The drawing under review shows one solid part. Ordinate dimensions are in mm from its lowest x, y, z. A direction names the side the tool comes from. Give positions to 0.01 mm unless a question says otherwise; leave off trailing zeros. Order: outer loops, then holes, each group sorted by start corner. A loop starts at its lowest first (then second) coordinate and runs counter-clockwise, first axis right, second up. Notation, with made-up numbers: (78, -23.5) -> (129, -23.5) arc R18 ccw to (129, -17.5) -> close; hole circle Ø9 at (79.5, 40). An arc over 180 degrees is marked (long way). Return JSON: item names as keys, results as strings. Group by question number.
1) For the marked faces 1, 2 and 3, list the 3-axis set-ups (+Z, -Z, +X, -X, +Y, -Y) from which the entire face can be reached by the end or side of a thin tool; tool diameter is ignored.
2) To check wall thickness, follow line 1 along X through (y, z) = (6.5, 33); line 2 along X through (y, z) = (16, 32); line 3 along Y through (x, z) = (53, 24). State the ranges of each line that lie inside material, in increasing order.
3) Add section B-B (x = 33). State how many separate pieces and enclosed holes the cut face has, then the cut area to 3 significant figures.
4) Add section A-A (y = 6.5). Give the boundary of the cut face in (x, z).
5) Insertion check: P1, Ø2, axis at y = 21, z = 51.5, coming from the +X side; P2, Ø6, axis at x = 55, y = 16.5, coming from the -Z side; P3, Ø6, axis at x = 41.5, y = 10.5, coming from the +Z side. Each pin has a flat end and moves straight along its axis. Give the tip position at first contact, or say it passes through.
6) The part is to be moulded in two halves that separate along X. For the marked faces 4, 5 and 6, say which applies: released by +X, released by -X, zero draft, split by the parting line, or undercut.
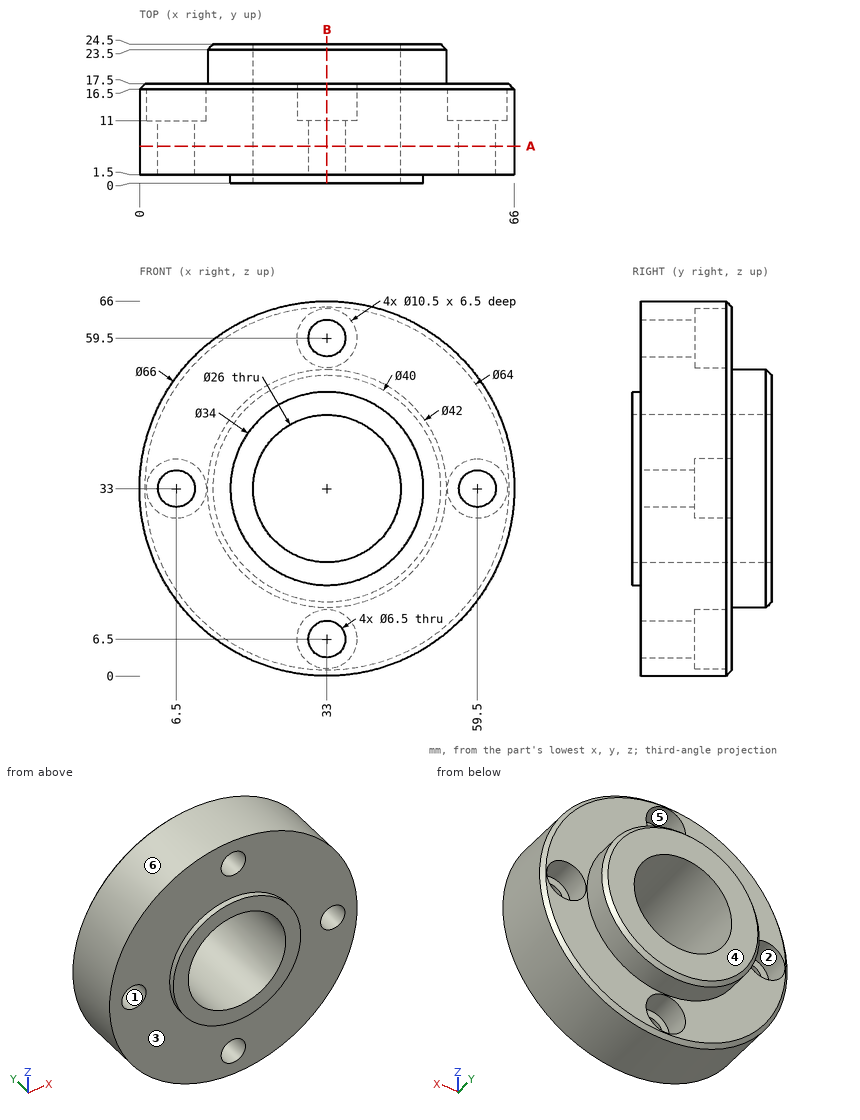
Evaluation:
{
 "1": {"face 1": "+Y, -Y", "face 2": "+Y", "face 3": "-Y"},
 "2": {"line 1": "0 to 3.25, 9.75 to 20, 46 to 56.25, 62.75 to 66", "line 2": "0.02 to 1.35, 11.65 to 20.04, 45.96 to 54.35, 64.65 to 65.98", "line 3": "1.5 to 17.5"},
 "3": {"separate pieces": "4", "enclosed holes": "0", "area": "502 mm^2"},
 "4": {"outline": "circle Ø66 at (33, 33); hole circle Ø6.5 at (6.5, 33); hole circle Ø26 at (33, 33); hole circle Ø6.5 at (33, 6.5); hole circle Ø6.5 at (33, 59.5); hole circle Ø6.5 at (59.5, 33)"},
 "5": {"P1": "x = 44.61", "P2": "z = 6.02", "P3": "z = 65.54"},
 "6": {"face 4": "zero draft", "face 5": "undercut", "face 6": "split by the parting line"}
}
